from build123d import *

# Parameters (mm, degrees)
PLACA_START              = -40.5
SK_PLACA_W               = 50
SK_PLACA_H               = 36
PLACA_DEPTH              = 6
EXTREMO_START            = -40.5
SK_EXTREMO_R             = 25
EXTREMO_DEPTH            = 6
ALOJAMIENTO_696ZZ_START  = -39.5
SK_ALOJAMIENTO_696ZZ_R   = 7.475
ALOJAMIENTO_696ZZ_DEPTH  = 5
PASO_EXTRACTOR_START     = -40.5
SK_PASO_EXTRACTOR_R      = 4
PASO_EXTRACTOR_DEPTH     = 1
EXTENSION_PESTANAS_START = -40.5
SK_EXTENSION_PESTANAS_W  = 50
SK_EXTENSION_PESTANAS_H  = 19
EXTENSION_PESTANAS_DEPTH = 6
PASANTES_M4_REPISA_START = -40.5
SK_PASANTES_M4_REPISA_R  = 2.25
PASANTES_M4_REPISA_DEPTH = 6


with BuildPart() as part:
    # Sk_Placa → Placa (new body)
    with BuildSketch(Plane(origin=(0, 0, 0), x_dir=(1, 0, 0), z_dir=(0, 1, 0)).offset(PLACA_START)):
        with Locations((0, -508)):
            Rectangle(SK_PLACA_W, SK_PLACA_H)
    extrude(amount=PLACA_DEPTH)

    # Sk_Extremo → Extremo (add)
    with BuildSketch(Plane(origin=(0, 0, 0), x_dir=(1, 0, 0), z_dir=(0, 1, 0)).offset(EXTREMO_START)):
        with Locations((0, -490)):
            Circle(SK_EXTREMO_R)
    extrude(amount=EXTREMO_DEPTH)

    # Sk_Alojamiento_696ZZ → Alojamiento_696ZZ (cut)
    with BuildSketch(Plane(origin=(0, 0, 0), x_dir=(1, 0, 0), z_dir=(0, 1, 0)).offset(ALOJAMIENTO_696ZZ_START)):
        with Locations(Location((0, -490, 0), (0, 0, 270))):
            Circle(SK_ALOJAMIENTO_696ZZ_R)
    extrude(amount=ALOJAMIENTO_696ZZ_DEPTH, mode=Mode.SUBTRACT)

    # Sk_Paso_extractor → Paso_extractor (cut)
    with BuildSketch(Plane(origin=(0, 0, 0), x_dir=(1, 0, 0), z_dir=(0, 1, 0)).offset(PASO_EXTRACTOR_START)):
        with Locations(Location((0, -490, 0), (0, 0, 270))):
            Circle(SK_PASO_EXTRACTOR_R)
    extrude(amount=PASO_EXTRACTOR_DEPTH, mode=Mode.SUBTRACT)

    # Sk_Extension_pestanas → Extension_pestanas (add)
    with BuildSketch(Plane(origin=(0, 0, 0), x_dir=(1, 0, 0), z_dir=(0, 1, 0)).offset(EXTENSION_PESTANAS_START)):
        with Locations((0, -535.5)):
            Rectangle(SK_EXTENSION_PESTANAS_W, SK_EXTENSION_PESTANAS_H)
    extrude(amount=EXTENSION_PESTANAS_DEPTH)

    # Sk_Pasantes_M4_repisa → Pasantes_M4_repisa (cut)
    with BuildSketch(Plane(origin=(0, 0, 0), x_dir=(1, 0, 0), z_dir=(0, 1, 0)).offset(PASANTES_M4_REPISA_START)):
        with Locations(Location((-15, -534, 0), (0, 0, 270))):
            Circle(SK_PASANTES_M4_REPISA_R)
        with Locations(Location((15, -534, 0), (0, 0, 270))):
            Circle(SK_PASANTES_M4_REPISA_R)
    extrude(amount=PASANTES_M4_REPISA_DEPTH, mode=Mode.SUBTRACT)


solid = part.part
Can you work these out from the model? Positions are in its coordinate system, mm. A direction names the side the tool comes from. Give positions to 0.01 mm unless a question says otherwise; leave off trailing zeros. Loops run counter-clockwise (first coordinate to the right, second up) from the corner with the lowest first, then second, coordinate; pieces in that order, holes last. Notation, with made-up numbers: (76, -4) - (132, -4) arc R13 cw to (132, 5) - close; hole circle Ø5 at (-5.5, 39). An arc over 180 degrees is marked (long way). Answer as a JSON object with one key per item and string values.
Q1. Imagine slicing it at D-D on x = -20. Write out the boundary of the cut face in (y, z).
Geometry says:
{"outline": "(-40.5, 475) - (-34.5, 475) - (-34.5, 545) - (-40.5, 545) - close"}
Q2. Which directions (+Z, -Z, +X, -X, +Y, -Y) give clear straight access to the entire face, cutting with the end or side of a thin tool? Please do faces 4 (the flat face through (0, -34.5, 504)), 5 (the cylindrical face through (0.329, -37.035, 482.532)).
Geometry says:
{"face 4": "+Z, -Z, +X, -X, +Y", "face 5": "+Y"}
Q3. Will these pins go through, and if not, where does the flat tip stop? P1, Ø4.5, axis at x = 3.5, z = 486.5, coming from the +Y side; P2, Ø2, axis at y = -35.5, z = 473.5, coming from the +X side; P3, Ø6, axis at x = -15, z = 534, coming from the +Y side; P4, Ø2, axis at x = -5, y = -36, coming from the -Z side.
Geometry says:
{"P1": "y = -39.5", "P2": "x = 19.62", "P3": "y = -34.5", "P4": "z = 465.32"}
Q4. If I drill on L1, parallel to X at y = -36.15, z = 534; L2, parallel to X at y = -37.75, z = 490 (3 decimals); L3, parallel to X at y = -40, z = 490, over which ranges is the centre line in solid material (lowest first)?
Geometry says:
{"L1": "-25 to -17.25, -12.75 to 12.75, 17.25 to 25", "L2": "-25 to -7.475, 7.475 to 25", "L3": "-25 to -4, 4 to 25"}
Q5. Imagine slicing it at C-C on z = 491.5. Write out the boundary of the cut face in (x, y), plus the area to 3 significant figures.
Geometry says:
{"outline": "(-25, -40.5) - (-3.71, -40.5) - (-3.71, -39.5) - (-7.32, -39.5) - (-7.32, -34.5) - (-25, -34.5) - close; (3.71, -40.5) - (25, -40.5) - (25, -34.5) - (7.32, -34.5) - (7.32, -39.5) - (3.71, -39.5) - close", "area": "219 mm²"}
Q6. Imagine slicing it at B-B on y = -36.35. Write out the boundary of the cut face in (x, z) (3 decimals).
Geometry says:
{"outline": "(-25, 490) arc R25 ccw to (25, 490) - (25, 545) - (-25, 545) - close; hole circle Ø4.5 at (-15, 534); hole circle Ø14.95 at (0, 490); hole circle Ø4.5 at (15, 534)"}
Q7. If we mould it in two halves opening along Z, with no side actions, what happens to faces 1 (the cylindrical face through (0, -40, 486)), 2 (the cylindrical face through (0.55, -37.542, 465.006)), 3 (the flat face through (-25, -38, 518))? For each: pulls with the +Z half, pulls with the -Z half, needs draft (parallel to the pull), parting line crosses it, or undercut.
Geometry says:
{"face 1": "undercut", "face 2": "pulls with the -Z half", "face 3": "needs draft"}
Q8. Imagine slicing it at A-A on x = 0. Write out the boundary of the cut face in (y, z) (3 decimals), plus the area to 3 significant figures.
Geometry says:
{"outline": "(-40.5, 465) - (-34.5, 465) - (-34.5, 482.525) - (-39.5, 482.525) - (-39.5, 486) - (-40.5, 486) - close; (-40.5, 494) - (-39.5, 494) - (-39.5, 497.475) - (-34.5, 497.475) - (-34.5, 545) - (-40.5, 545) - close", "area": "397 mm²"}
